```python
from build123d import *

# Parameters (mm, degrees)
BOSS_EXTRUDE1_DEPTH   = 16.5
M10_CLEARANCE_HOLE1_D = 11.8125


with BuildPart() as part:
    # Sketch1 → Boss-Extrude1 (new body)
    with BuildSketch(Plane.XY.offset(8.25)):
        Polygon((22.406299796, -1.906250123), (5.308030128, 8.36411953), (3.061199903, 9.42140007), (0.622018993, 9.886699677), (-1.856250048, 9.730779648), (-4.217879772, 8.963439941), (-22.406200409, -1.90625), (-22.406200409, -5.90625), (22.406299796, -5.90625), align=None)
    extrude(amount=-BOSS_EXTRUDE1_DEPTH)

    # Sketch2 → Cut-Revolve1 (revolve, cut)
    with BuildSketch(Plane.XY, mode=Mode.PRIVATE) as cut_revolve1_sk:
        Polygon((26.531393942, 8.080018406), (16.1562, 8.080018406), (16.1562, -5.90625), (18.4062, -5.90625), (18.4062, -3.70625), (22.4062, -3.70625), align=None)
    revolve(cut_revolve1_sk.sketch.rotate(Axis((16.1562, 8.080018406, 0), (0, -1, 0)), 92.019039349), axis=Axis((16.1562, 8.080018406, 0), (0, -1, 0)), mode=Mode.SUBTRACT)

    # Sketch3 → Cut-Revolve2 (revolve, cut)
    with BuildSketch(Plane(origin=(0, 0, 0), x_dir=(-1, 0, 0), z_dir=(0, 0, -1)), mode=Mode.PRIVATE) as cut_revolve2_sk:
        Polygon((13.9062, -5.90625), (16.1562, -5.90625), (16.1562, 8.015867372), (5.80345892, 8.015867372), (9.9062, -3.70625), (13.9062, -3.70625), align=None)
    revolve(cut_revolve2_sk.sketch.rotate(Axis((-16.1562, -5.90625, 0), (0, 1, 0)), 270), axis=Axis((-16.1562, -5.90625, 0), (0, 1, 0)), mode=Mode.SUBTRACT)

    # M10 Clearance Hole1 (through all)
    with Locations(Plane.XY.offset(8.25)):
        with Locations((0, -0.02)):
            Hole(M10_CLEARANCE_HOLE1_D / 2)


solid = part.part
```
CAD build for the part. Positions are in the model's coordinates, mm. A direction names the side the tool comes from. Round coordinates to 2 decimals unless told otherwise and drop trailing zeros. Order: outer loops, then holes, each group sorted by start corner. A loop starts at its lowest first (then second) coordinate and runs counter-clockwise, first axis right, second up. Notation, with made-up numbers: (46, 6.5) - (62, 6.5) arc R35 ccw to (62, 39.5) - close; hole circle Ø10 at (63.5, 22.25). An arc over 180 degrees is marked (long way). Use CSV: the item, a comma, the result in double quotes. Start each with the question number.
1) Wall check: L1, parallel to Z at x = 16, y = -4.25; L2, parallel to X at y = -5.2, z = 0; L3, parallel to X at y = -5.1, z = 0. Give the ranges that are in metal, low to high. Write a range as [from, to].
2) Pin check, flat tips, straight feed: pin 1 Ø5 at (x, z) = (-16.16, 0) entering from +Y; pin 2 Ø1 at (y, z) = (-1, 2.5) entering from -X; pin 3 Ø1 at (x, y) = (13.5, 5.5) entering from +Z. Stop position of each tip, or through.
3) Tool access for faces 1 (the flat face through (-5.61, 8.13, 0.12)), 2 (the flat face through (-16, -3.706, 3)): list every direction of +Z, -Z, +X, -X, +Y, -Y with a clear straight run to the whole face (end or side of a thin tool).
4) Saw through at D-D (y = -0.02). List the corners of the cut face in (x, z), and give its area (3 significant figures).
5) Saw through at A-A (y = -4.5). List the corners of the cut face in (x, z), and give its area (3 significant figures).
6) Two-plate mould, pull along Y, no slides. Class faces 3 (the cylindrical face through (-0.25, 5.88, -0.12)), 4 (the flat face through (11, -5.906, 0)), 5 (the flat face through (-20.806, -0.95, -6.944)): pulls with the +Y half, pulls with the -Y half, needs draft (parallel to the pull), parting line crosses it, or undercut.
7) Saw through at C-C (x = -1). List the corners of the cut face in (y, z).
8) Saw through at B-B (y = 5.25). List the corners of the cut face in (x, z), and give its area (3 significant figures).
Values follow:
1,L1,"z = [-8.25, -2.24], [2.24, 8.25]"
1,L2,"x = [-22.41, -18.41], [-13.91, -2.84], [2.84, 13.91], [18.41, 22.41]"
1,L3,"x = [-22.41, -18.41], [-13.91, -3.01], [3.01, 13.91], [18.41, 22.41]"
2,pin 1,"stops at y = -3.71"
2,pin 2,"stops at x = -9.68"
2,pin 3,"passes through"
3,face 1,"+Z, -Z, -X, +Y"
3,face 2,"+Y"
4,outline,"(-19.25, -8.25) - (-5.91, -8.25) - (-5.91, 8.25) - (-19.25, 8.25) - (-19.25, 6.88) arc R7.54 cw (long way) to (-19.25, -6.88) - close; (5.91, -8.25) - (19.27, -8.25) - (19.27, -6.87) arc R7.54 cw (long way) to (19.27, 6.87) - (19.27, 8.25) - (5.91, 8.25) - close"
4,area,"171 mm2"
5,outline,"(-22.41, -8.25) - (-3.85, -8.25) - (-3.85, 8.25) - (-22.41, 8.25) - close; (3.85, -8.25) - (22.41, -8.25) - (22.41, 8.25) - (3.85, 8.25) - close; hole circle Ø4.5 at (-16.16, 0); hole circle Ø4.5 at (16.16, 0)"
5,area,"581 mm2"
6,face 3,"undercut"
6,face 4,"pulls with the -Y half"
6,face 5,"pulls with the +Y half"
7,outline,"(-5.91, -8.25) - (-5.84, -8.25) - (-5.84, 8.25) - (-5.91, 8.25) - close; (5.8, -8.25) - (9.78, -8.25) - (9.78, 8.25) - (5.8, 8.25) - close"
8,outline,"(-10.43, -8.25) - (-2.67, -8.25) - (-2.67, 8.25) - (-10.43, 8.25) - (-10.43, 7.44) arc R9.38 cw to (-10.43, -7.44) - close; (2.67, -8.25) - (10.49, -8.25) - (10.49, -7.48) arc R9.38 cw to (10.49, 7.48) - (10.49, 8.25) - (2.67, 8.25) - close"
8,area,"180 mm2"
